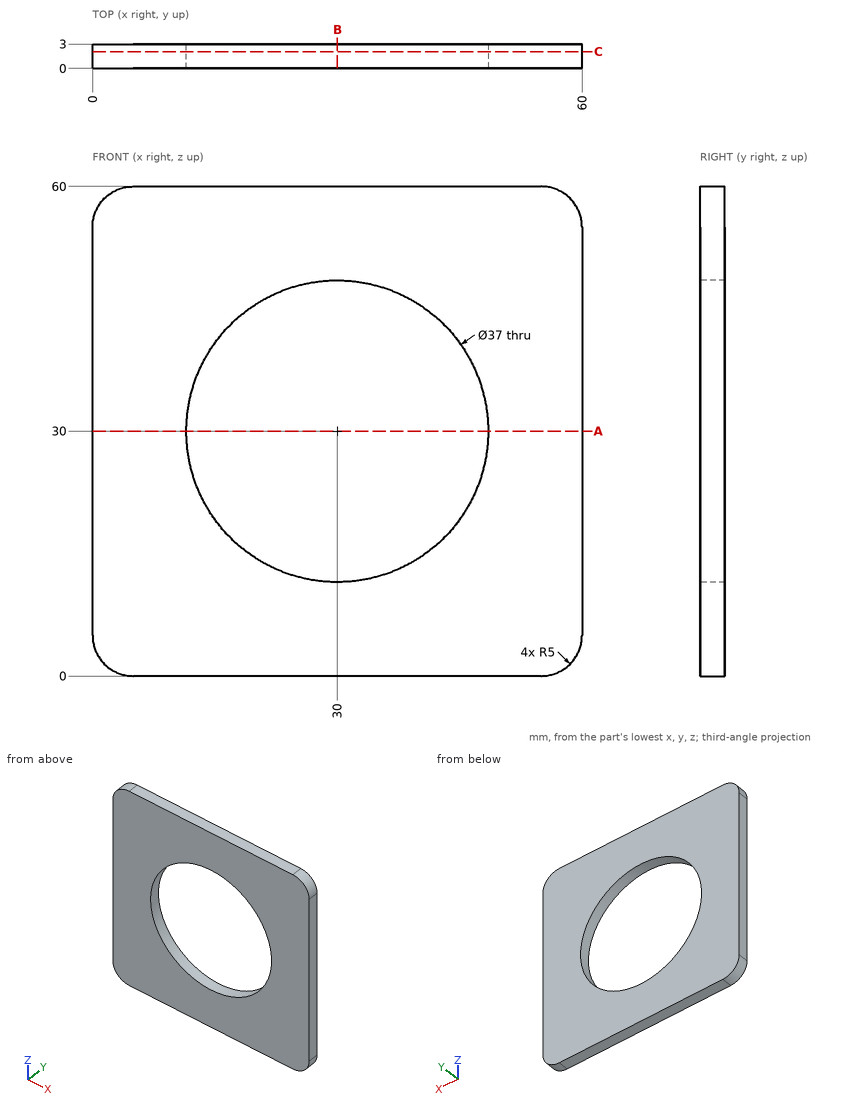
Geometry check sheet. Reference: drawing and pictorial views, mm from the part's lowest x, y, z. Give positions to 0.01 mm unless a question says otherwise; leave off trailing zeros. Order: outer loops, then holes, each group sorted by start corner. A loop starts at its lowest first (then second) coordinate and runs counter-clockwise, first axis right, second up. Notation, with made-up numbers: M -10,1 L -1,1 A12 cw -1,19 Z; hole C 31,-27.5 d8. An arc over 180 degrees is marked long. Answer in a Markdown table with one row per item. Add a question column.
Q1. Sectioned sample at B-B, the plane x = 30. Record the boundary of the cut face in (y, z), and give its area (3 significant figures).
Q2. Sectioned sample at C-C, the plane y = 2.05. Record the boundary of the cut face in (x, z), and give its area (3 significant figures).
Q3. Thickness scan on L1, parallel to Z at x = 30, y = 1.2; L2, parallel to X at y = 0.15, z = 25.5; L3, parallel to X at y = 0.95, z = 21. Record the ranges inside material, lowest first.
Q4. Sectioned sample at A-A, the plane z = 30. Record the boundary of the cut face in (x, y).
Verdict:
| question | item | result |
|---|---|---|
| 1 | outline | M 0,0 L 3,0 L 3,11.5 L 0,11.5 Z; M 0,48.5 L 3,48.5 L 3,60 L 0,60 Z |
| 1 | area | 69.0 mm² |
| 2 | outline | M 0,5 A5 ccw 5,0 L 55,0 A5 ccw 60,5 L 60,55 A5 ccw 55,60 L 5,60 A5 ccw 0,55 Z; hole C 30,30 d37 |
| 2 | area | 2,500 mm² |
| 3 | L1 | 0 to 11.5, 48.5 to 60 |
| 3 | L2 | 0 to 12.06, 47.94 to 60 |
| 3 | L3 | 0 to 13.84, 46.16 to 60 |
| 4 | outline | M 0,0 L 11.5,0 L 11.5,3 L 0,3 Z; M 48.5,0 L 60,0 L 60,3 L 48.5,3 Z |
